Input: part model. Units: mm. Frame: model coordinates. A direction names the side the tool comes from. Coordinates: 2 decimals unless noted, no trailing zeros. Loops run counter-clockwise (first coordinate to the right, second up) from the corner with the lowest first, then second, coordinate; pieces in that order, holes last.
Item 1: Section C-C on x = -15.5. Return loops of the section in (y, z), and give its area (3 significant figures).
Item 2: Section A-A on z = 0. Return loops of the section in (x, y), and give its area (3 significant figures).
Item 3: Ray query, line 1 along X through (y, z) = (1.65, 0); line 2 along Y through (x, z) = (19, 5); line 3 along Z through (x, y) = (0, 1.25). Return the intervals inside material, ascending.
Item 4: Reachability of faces 4 (the flat face through (-5, 0, 18)), 5 (the flat face through (-15, 2, -13.092)), 6 (the cylindrical face through (-20.372, 6.944, 18.278)) from +Z, -Z, +X, -X, +Y, -Y: full face, straight path, thin tool, end or side. Return the list, or none.
Item 5: Section D-D on y = 8. Return loops of the section in (x, z), and give its area (3 significant figures).
Item 6: Section B-B on y = 1.25. Return loops of the section in (x, z).
Item 7: Contact query for flat-ended pins moving along their axis: P1, Ø5, axis at y = 7, z = 5.5, coming from the +X side; P2, Ø6, axis at x = 0, y = 3.5, coming from the +Z side; P3, Ø2.5, axis at x = -15, y = 1.5, coming from the -Z side; P4, Ø5, axis at y = 8.5, z = -15.5, coming from the -X side. Output: stop coordinate, or through.
Item 8: Pull-direction query (Z, two-part tool) for faces 1 (the cylindrical face through (17.277, 6.944, -17.569)), 2 (the flat face through (20, 1, -27.6)), 3 (the flat face through (-23, 1, 0)); classes: released by +Z, released by -Z, zero draft, split by the parting line, or undercut.
```python
from build123d import *

# Parameters (mm, degrees)
SKETCH1_W           = 46
SKETCH1_H           = 55.2
BOSS_EXTRUDE1_DEPTH = 3
SKETCH4_W           = 33.02335113
SKETCH4_H           = 20.828153407
CUT_EXTRUDE1_DEPTH  = 8
SKETCH3_R           = 17.9
CUT_EXTRUDE2_DEPTH  = 8
SKETCH5_R           = 1.25
BOSS_EXTRUDE2_DEPTH = 8


with BuildPart() as part:
    # Sketch1 → Boss-Extrude1 (new body)
    with BuildSketch(Plane(origin=(0, 0, 0), x_dir=(1, 0, 0), z_dir=(0, 1, 0))):
        Rectangle(SKETCH1_W, SKETCH1_H)
    extrude(amount=BOSS_EXTRUDE1_DEPTH)

    # Sketch4 → Cut-Extrude1 (cut)
    with BuildSketch(Plane(origin=(0, 3, 0), x_dir=(1, 0, 0), z_dir=(0, 1, 0))):
        with Locations((-0.224140392, 23.506208916)):
            Rectangle(SKETCH4_W, SKETCH4_H)
    extrude(amount=-CUT_EXTRUDE1_DEPTH, mode=Mode.SUBTRACT)

    # Sketch3 → Cut-Extrude2 (cut)
    with BuildSketch(Plane(origin=(0, 3, 0), x_dir=(1, 0, 0), z_dir=(0, 1, 0))):
        Circle(SKETCH3_R)
    extrude(amount=-CUT_EXTRUDE2_DEPTH, mode=Mode.SUBTRACT)

    # Sketch5 → Boss-Extrude2 (add)
    with BuildSketch(Plane(origin=(0, 3, 0), x_dir=(1, 0, 0), z_dir=(0, 1, 0))):
        with Locations(Location((-19.317913276, 18.489975821, 0), (0, 0, 90))):
            Circle(SKETCH5_R)
        with Locations(Location((18.122086724, 18.489975821, 0), (0, 0, 90))):
            Circle(SKETCH5_R)
        with Locations(Location((-19.317913276, -18.950024179, 0), (0, 0, 90))):
            Circle(SKETCH5_R)
        with Locations(Location((18.084134894, -18.924464602, 0), (0, 0, 90))):
            Circle(SKETCH5_R)
    extrude(amount=BOSS_EXTRUDE2_DEPTH)


solid = part.part
```
Results found:
1. outline: (0, -13.09) - (3, -13.09) - (3, -8.95) - (0, -8.95) - close; (0, 8.95) - (3, 8.95) - (3, 27.6) - (0, 27.6) - close
1. area: 68.4 mm2
2. outline: (-23, 0) - (-17.9, 0) - (-17.9, 3) - (-23, 3) - close; (17.9, 0) - (23, 0) - (23, 3) - (17.9, 3) - close
2. area: 30.6 mm2
3. line 1: x = -23 to -17.9, 17.9 to 23
3. line 2: y = 0 to 3
3. line 3: z = 17.9 to 27.6
4. face 4: +Z, -Z, +X, -X, -Y
4. face 5: -Z, +Y, -Y
4. face 6: +Y
5. outline: circle Ø2.5 at (-19.32, -18.49); circle Ø2.5 at (-19.32, 18.95); circle Ø2.5 at (18.08, 18.92); circle Ø2.5 at (18.12, -18.49)
5. area: 19.6 mm2
6. outline: (-23, -27.6) - (-16.74, -27.6) - (-16.74, -13.09) - (-12.21, -13.09) arc R17.9 cw (long way) to (12.21, -13.09) - (16.29, -13.09) - (16.29, -27.6) - (23, -27.6) - (23, 27.6) - (-23, 27.6) - close
7. P1: passes through
7. P2: stops at z = 27.6
7. P3: stops at z = -13.09
7. P4: stops at x = -20.47
8. face 1: undercut
8. face 2: released by -Z
8. face 3: zero draft
